```python
from build123d import *

# Parameters (mm, degrees)
F2_DEPTH       = 2
F2_DEPTH_BACK  = 2
F3_ANGLE       = 45
F4_ANGLE       = 45
F5_ANGLE       = 45
F10_DEPTH      = 0.5
F12_DEPTH      = 0.5
F15_DEPTH      = 0.5
F18_DEPTH      = 0.5
F19_R          = 1.25
F20_DEPTH      = 22.501
F20_DEPTH_BACK = 22.501


with BuildPart() as f2:
    # F1 (on Top) → F2 (new body, two sides)
    with BuildSketch(Plane.XY) as f2_sk:
        Polygon((22.5, 0), (-22.5, 0), (0, -38.9711431703), align=None)
    extrude(amount=F2_DEPTH)
    extrude(f2_sk.sketch, amount=-F2_DEPTH_BACK)


with BuildPart() as f3_1:
    # F3: copy of F2
    add(f2.part.rotate(Axis((0, -18.774760887, 0), (0, 1, 0)), F3_ANGLE))


with BuildPart() as f4_1:
    # F4: copy of F3_1
    add(f3_1.part.rotate(Axis((0, -18.774760887, 0), (0, 1, 0)), F4_ANGLE))


with BuildPart() as f5_1:
    # F5: copy of F4_1
    add(f4_1.part.rotate(Axis((0, -18.774760887, 0), (0, 1, 0)), F5_ANGLE))


with BuildPart() as f2_1:
    add(f2.part)

    # F6: union F3_1, F4_1, F5_1
    add(f3_1.part)
    add(f4_1.part)
    add(f5_1.part)

    # F9 (on line) → F10 (cut, symmetric)
    with BuildSketch(Plane(origin=(0, 0, 0), x_dir=(0, -1, 0), z_dir=(-0.7071067812, 0, 0.7071067812))):
        Polygon((0, -20.1905989232), (20, -8.6435935394), (20, 8.6435935394), (0, 20.1905989232), align=None)
    extrude(amount=F10_DEPTH, both=True, mode=Mode.SUBTRACT)

    # F11 (on Right) → F12 (cut, symmetric)
    with BuildSketch(Plane.YZ):
        Polygon((-20, -8.6435935394), (0, -20.1905989232), (0, 20.1905989232), (-20, 8.6435935394), align=None)
    extrude(amount=F12_DEPTH, both=True, mode=Mode.SUBTRACT)

    # F14 (on Top) → F15 (cut, symmetric)
    with BuildSketch(Plane.XY):
        Polygon((20.1905989232, 0), (-20.1905989232, 0), (-8.6435935394, -20), (8.6435935394, -20), align=None)
    extrude(amount=F15_DEPTH, both=True, mode=Mode.SUBTRACT)

    # F16 (on Top) → F17 (revolve, cut)
    with BuildSketch(Plane.XY):
        with BuildLine():
            Line((47.749247402, 0), (22.5, 0))
            Line((22.5, 0), (0.4330127019, -38.2211431703))
            ThreePointArc((0.4330127019, -38.2211431703), (0.25, -38.4041558722), (0, -38.4711431703))
            Line((0, -38.4711431703), (0, -38.9711431703))
            Line((0, -38.9711431703), (0, -40.9711431703))
            Line((0, -40.9711431703), (49.3083149195, -40.9711431703))
            Line((49.3083149195, -40.9711431703), (47.749247402, 0))
        make_face()
    revolve(axis=Axis((0, -18.774760887, 0), (0, 1, 0)), mode=Mode.SUBTRACT)

    # F13 (on line) → F18 (cut, symmetric)
    with BuildSketch(Plane(origin=(0, 0, 0), x_dir=(0.7071067812, 0, -0.7071067812), z_dir=(-0.7071067812, 0, -0.7071067812))):
        Polygon((-20.1905989232, 0), (20.1905989232, 0), (8.6435935394, 20), (-8.6435935394, 20), align=None)
    extrude(amount=F18_DEPTH, both=True, mode=Mode.SUBTRACT)

    # F19 (on Top) → F20 (cut, two sides)
    with BuildSketch(Plane.XY) as f20_sk:
        with Locations((0, -33.7211431703)):
            Circle(F19_R)
    extrude(amount=-F20_DEPTH, mode=Mode.SUBTRACT)
    extrude(f20_sk.sketch, amount=F20_DEPTH_BACK, mode=Mode.SUBTRACT)


solid = f2_1.part
```
Verification items for the finished model (mm, model axes). Round coordinates to 2 decimals unless told otherwise and drop trailing zeros. Write each loop counter-clockwise with the first axis right and the second up, starting at its lowest first coordinate (ties: lowest second). Pieces come first, ordered by that corner, then holes. Notation, with made-up numbers: (87, -5.75) -> (94, -5.75) arc R17 cw to (94, 19.25) -> close; hole circle Ø11 at (45, 52.5). An arc over 180 degrees is marked (long way). Write each question's results on one line, items separated by ' | '. Start each with the question number.
1. Depth check by flat-ended pin: P1, Ø5.5, axis at x = 13, y = -13, coming from the +Z side; P2, Ø9.5, axis at y = -12.5, z = -8.5, coming from the -X side; P3, Ø8, axis at x = -5, z = -2.5, coming from the +Y side; P4, Ø3, axis at x = 3, y = -8, coming from the +Z side. Enter the tip coordinate at first touch or a pass-through.
2. Cross-section at A-A (y = -21). Enter the section's corners in (x, z), then the cut area to 3 significant figures.
3. Draft check along Z on faces 1 (the flat face through (-1, 0, 3)), 2 (the conical face through (-4.723, -27.872, -4.331)), 3 (the flat face through (12, -11, -2)). Enter one of: +Z half, -Z half, draft (parallel to the pull), parting line (faces both ways), or undercut.
Solutions:
1) P1: stops at z = 11.74 | P2: stops at x = -13.8 | P3: stops at y = 0 | P4: stops at z = 18.42
2) outline: (-10.18, -2) -> (-4.83, -2) -> (-8.61, -5.78) arc R10.38 ccw to (-5.78, -8.61) -> (-2, -4.83) -> (-2, -10.18) arc R10.38 ccw to (2, -10.18) -> (2, -4.83) -> (5.78, -8.61) arc R10.38 ccw to (8.61, -5.78) -> (4.83, -2) -> (10.18, -2) arc R10.38 ccw to (10.18, 2) -> (4.83, 2) -> (8.61, 5.78) arc R10.38 ccw to (5.78, 8.61) -> (2, 4.83) -> (2, 10.18) arc R10.38 ccw to (-2, 10.18) -> (-2, 4.83) -> (-5.78, 8.61) arc R10.38 ccw to (-8.61, 5.78) -> (-4.83, 2) -> (-10.18, 2) arc R10.38 ccw to start | area: 253 mm2
3) face 1: draft | face 2: parting line | face 3: undercut
